from build123d import *

# Parameters (mm, degrees)
SKETCH1_W                        = 44.45
SKETCH1_H                        = 44.45
SKETCH1_W_2                      = 38.1
SKETCH1_H_2                      = 38.1
BOSS_EXTRUDE1_DEPTH              = 1984.375
F_17_64_0_26563_DIAMETER_HOLE1_D = 6.747002


with BuildPart() as part:
    # Sketch1 → Boss-Extrude1 (new body)
    with BuildSketch(Plane(origin=(0, 0, 0), x_dir=(1, 0, 0), z_dir=(0, 1, 0))):
        Rectangle(SKETCH1_W, SKETCH1_H)
        Rectangle(SKETCH1_W_2, SKETCH1_H_2, mode=Mode.SUBTRACT)
    extrude(amount=BOSS_EXTRUDE1_DEPTH)

    # 17/64 (0.26563) Diameter Hole1 (through all)
    with Locations(Plane.XY.offset(22.225)):
        with Locations((0, 812.8), (0, 120.65), (0, 1171.575), (0, 1863.725)):
            Hole(F_17_64_0_26563_DIAMETER_HOLE1_D / 2)


solid = part.part
Input: part model. Units: mm. Frame: model coordinates. A direction names the side the tool comes from. Give positions to 0.01 mm unless a question says otherwise; leave off trailing zeros. Write each loop counter-clockwise with the first axis right and the second up, starting at its lowest first coordinate (ties: lowest second). Pieces come first, ordered by that corner, then holes.
Q1. Pull-direction query (X, two-part tool) for faces 1 (the face through (-22.225, 978, 0)), 2 (the face through (19.4, 0, -0.3)), 3 (the face through (0, 978, 19.05)), 4 (the face through (19.05, 978, 0)); classes: pulls with the +X half, pulls with the -X half, needs draft (parallel to the pull), parting line crosses it, or undercut.
Q2. First-contact query: P1, Ø5.5, axis at x = 0, y = 812.8, coming from the +Z side. Flat tip, straight axial feed; report the tip coordinate or a pass-through.
Q3. Section A-A, the plane z = 11.5. Output: boundary loops of the cut face in (x, y) (3 decimals), plus the area to 3 significant figures.
Q4. Material intervals for probe 1 along Y at (x, z) = (0, 20.75) (1 decimal); probe 2 along X at (y, z) = (812.8, 19.8) (1 decimal); probe 3 along Z at (x, y) = (12.5, 227.5) (3 decimals), sorted ascending.
Q5. Section B-B, the plane y = 1328.5. Output: boundary loops of the cut face in (x, z) (3 decimals), plus the area to 3 significant figures.
Q6. Set-up query: faces 5 (the face through (0, 978, 22.225)), 6 (the face through (0, 978, -19.05)). Return all of +Z, -Z, +X, -X, +Y, -Y with unobstructed straight access to the full face (end or side cutting, diameter ignored); none if empty.
Filled in:
1. face 1: pulls with the -X half
1. face 2: needs draft
1. face 3: undercut
1. face 4: undercut
2. P1: passes through
3. outline: (-22.225, 0) - (-19.05, 0) - (-19.05, 1984.375) - (-22.225, 1984.375) - close; (19.05, 0) - (22.225, 0) - (22.225, 1984.375) - (19.05, 1984.375) - close
3. area: 12,600 mm2
4. probe 1: y = 0 to 117.3, 124 to 809.4, 816.2 to 1168.2, 1174.9 to 1860.4, 1867.1 to 1984.4
4. probe 2: x = -22.2 to -3.4, 3.4 to 22.2
4. probe 3: z = -22.225 to -19.05, 19.05 to 22.225
5. outline: (-22.225, -22.225) - (22.225, -22.225) - (22.225, 22.225) - (-22.225, 22.225) - close; hole (-19.05, -19.05) - (19.05, -19.05) - (19.05, 19.05) - (-19.05, 19.05) - close
5. area: 524 mm2
6. face 5: +Z, +X, -X, +Y, -Y
6. face 6: +Y, -Y
